Work out the finished part from the listing and answer in its coordinate system (mm). Face numbers are marked on the shaded views. A direction names the side the tool comes from. Coordinates: 2 decimals unless noted, no trailing zeros. Order: outer loops, then holes, each group sorted by start corner. A loop starts at its lowest first (then second) coordinate and runs counter-clockwise, first axis right, second up. Notation, with made-up numbers: (59, 50.25) -> (106, 50.25) arc R37 ccw to (106, 89.25) -> close; hole circle Ø3 at (-36.5, -6.5). An arc over 180 degrees is marked (long way). Use one line per item in the form item = value.
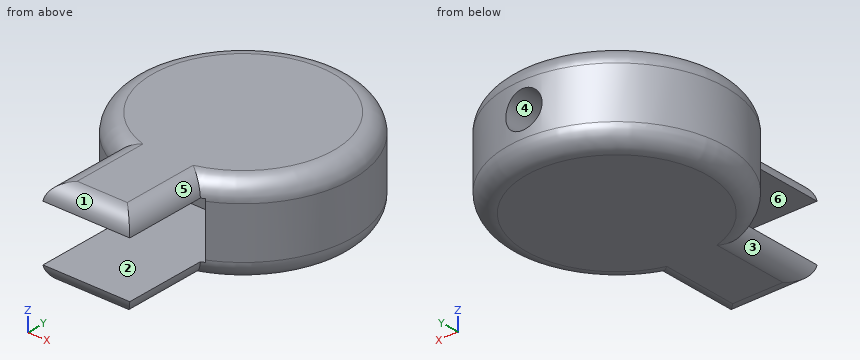
from build123d import *

# Parameters (mm, degrees)
F1_DEPTH = 12.1
F2_R     = 2.53999
F3_W     = 13.0256410256
F3_H     = 7.62
F4_DEPTH = 20
F5_R     = 2.5
F6_DEPTH = 25.4


# Not quite as in the source:
# - a fillet or chamfer is up to 0.001 mm smaller than in the source, because OpenCascade refuses the exact size


with BuildPart() as f1:
    # F0 (on Top) → F1 (new body)
    with BuildSketch(Plane.XY):
        with BuildLine():
            Line((6, -25), (6, -13.7477270849))
            ThreePointArc((6, -13.7477270849), (0, 15), (-6, -13.7477270849))
            Line((-6, -13.7477270849), (-6, -25))
            Line((-6, -25), (0, -25))
            Line((0, -25), (6, -25))
        make_face()
    extrude(amount=F1_DEPTH)

    # F2 (radius 2.54 in the source; OpenCascade refuses exactly that, so slightly less here)
    f2_edges = [f1.edges().sort_by_distance(p)[0] for p in [
        (-6, -19.373864, 12.1),
        (0, -25, 12.1),
        (6, -19.373864, 12.1),
        (0, 15, 12.1),
        (-6, -19.373864, 0),
        (0, -25, 0),
        (6, -19.373864, 0),
        (0, 15, 0),
    ]]
    fillet(f2_edges, radius=F2_R)

    # F3 (on face) → F4 (cut)
    with BuildSketch(Plane.XZ.offset(25)):
        with Locations((0, 6.05)):
            Rectangle(F3_W, F3_H)
    extrude(amount=-F4_DEPTH, mode=Mode.SUBTRACT)

    # F5 (on face) → F6 (cut)
    with BuildSketch(Plane.XZ.offset(5)):
        with Locations((0, 6.05)):
            Circle(F5_R)
    extrude(amount=-F6_DEPTH, mode=Mode.SUBTRACT)


solid = f1.part
(1) Which of the six approach directions +Z, -Z, +X, -X, +Y, -Y give full straight-line access (tool end or side, diameter ignored) to the marked faces 4, 5 and 6?
Data:
face_4 = +Y, -Y
face_5 = +Z, +X, -Y
face_6 = -Y
(2) Section C-C on z = 4.5 is taken. Write down the section's boundary in (x, y).
Data:
outline = (-6.51, -13.51) -> (-6.51, -5) -> (-1.96, -5) -> (-1.96, 14.87) arc R15 ccw to start; (1.96, -5) -> (6.51, -5) -> (6.51, -13.51) arc R15 ccw to (1.96, 14.87) -> close
(3) Section A-A on y = -15 is taken. Write down the section's boundary in (x, z), plus the area to 3 significant figures.
Data:
outline = (-5.98, 2.24) arc R2.54 ccw to (-3.46, 0) -> (3.46, 0) arc R2.54 ccw to (5.98, 2.24) -> close; (-5.98, 9.86) -> (5.98, 9.86) arc R2.54 ccw to (3.46, 12.1) -> (-3.46, 12.1) arc R2.54 ccw to start
area = 48.2 mm²
(4) Each of these flat-tipped pins is pushed along its axis until it touches: P1, Ø2, axis at x = -8, z = 3, coming from the +Y side; P2, Ø4, axis at x = 2, z = 5.5, coming from the -Y side; P3, Ø6, axis at x = 0, z = 6.05, coming from the +Y side; P4, Ø4, axis at y = -8, z = 7, coming from the -X side. Where does it stop, or does it pass through?
Data:
P1 = 13.27
P2 = -5
P3 = 15
P4 = -13.75
(5) Section D-D on z = 1.25 is taken. Write down the section's boundary in (x, y), plus the area to 3 significant figures.
Data:
outline = (-5.65, -24.65) -> (5.65, -24.65) -> (5.65, -13.52) arc R14.65 ccw (long way) to (-5.65, -13.52) -> close
area = 791 mm²
(6) The mould has two halves that part along Z. Classify the marked faces 1, 2 and 3: released by +Z, released by -Z, zero draft, split by the parting line, or undercut.
Data:
face_1 = released by +Z
face_2 = undercut
face_3 = released by -Z
(7) Section B-B on x = 0 is taken. Write down the section's boundary in (y, z), plus the area to 3 significant figures.
Data:
outline = (-24.98, 2.24) arc R2.54 ccw to (-22.46, 0) -> (12.46, 0) arc R2.54 ccw to (15, 2.54) -> (15, 3.55) -> (-5, 3.55) -> (-5, 2.24) -> close; (-24.98, 9.86) -> (-5, 9.86) -> (-5, 8.55) -> (15, 8.55) -> (15, 9.56) arc R2.54 ccw to (12.46, 12.1) -> (-22.46, 12.1) arc R2.54 ccw to start
area = 226 mm²
(8) Straight lines are drawn through the part: line 1 along Z through (x, y) = (-3, -11); line 2 along Z through (x, y) = (0, 1); line 3 along X through (y, z) = (-0.25, 6.05). For each, find the intervals that lie inside material, in ascending order.
Data:
line_1 = 0 to 2.24, 9.86 to 12.1
line_2 = 0 to 3.55, 8.55 to 12.1
line_3 = -15 to -2.5, 2.5 to 15
